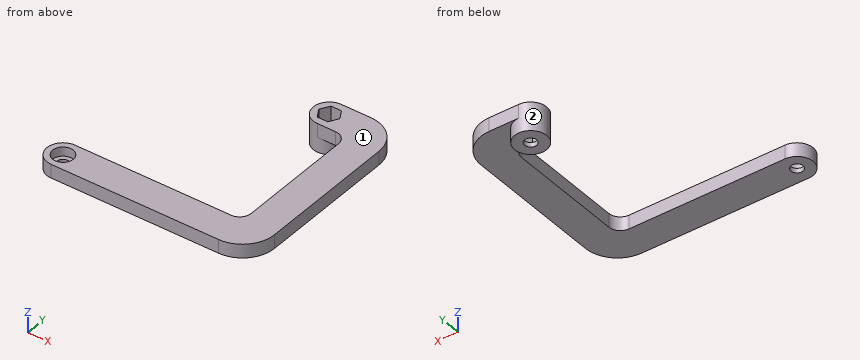
Autodesk Inventor part; units mm, degrees
ref_plane "YZ Plane" through (0, 0, 0) normal (1, 0, 0) x (0, 1, 0)
ref_plane "XZ Plane" through (0, 0, 0) normal (0, 1, 0) x (-1, 0, 0)
ref_plane "XY Plane" through (0, 0, 0) normal (0, 0, 1) x (1, 0, 0)
sketch "Skizze1" plane through (0, 0, 0) normal (0, 0, 1) x (1, 0, 0)
  circle A0 centre (0, 0) radius 2.5
  line L0 (0, 7) -> (13, 7)
  arc A1 (0, 7) -> (0, -7) centre (0, 0) ccw
  circle A2 centre (-60.334, -75) radius 2.5
  line L1 (-60.334, -68) -> (8, -68)
  line L2 (13, -63) -> (13, -12)
  line L3 (27, -7) -> (27, -68)
  line L4 (13, -82) -> (-60.334, -82)
  arc A3 (-60.334, -68) -> (-60.334, -82) centre (-60.334, -75) ccw
  line L5 (20, -82) -> (20, 7) construction
  line L6 (0, 0) -> (-60.334, -75) construction
  line L7 (-60.334, -75) -> (-110.6881, -137.5941) construction
  line L8 (-60.334, -75) -> (20, -75) construction
  circle A4 centre (-60.334, -75) radius 7
  arc A5 (27, -7) -> (13, 7) centre (13, -7) ccw
  arc A6 (13, -82) -> (27, -68) centre (13, -68) ccw
  arc A7 (8, -68) -> (13, -63) centre (8, -63) ccw
  arc A8 (13, -12) -> (8, -7) centre (8, -12) ccw
  circle A9 centre (0, 0) radius 7
  line L9 (8, -7) -> (0, -7)
  line L10 (-2.3094, -4) -> (-4.6188, 0)
  line L11 (-4.6188, 0) -> (-2.3094, 4)
  line L12 (-2.3094, 4) -> (2.3094, 4)
  line L13 (2.3094, 4) -> (4.6188, 0)
  line L14 (4.6188, 0) -> (2.3094, -4)
  line L15 (2.3094, -4) -> (-2.3094, -4)
  point P0 (-60.334, -68)
  point P1 (13, 7)
  point P2 (0, -7)
  point P3 (0, -7)
  dimension "d0" = 5
  dimension "d10" = 75
  dimension "d11" = 14
  dimension "d14" = 176.5899
  dimension "d19" = 20
  dimension "d20" = 7
  dimension "d25" = 5
  dimension "d26" = 14
  dimension "d41" = 8
extrude "Extrusion1" add sketch "Skizze1" along normal blind 6 contours A9 A1 | L0 A5 L3 A6 L4 A4 L1 A7 L2 A8 L9 A9 | A3 A4 | L10 L11 L12 L13 L14 L15
extrude "Extrusion2" add sketch "Skizze1" against normal blind 6.5 contours A9 A1 | L10 L11 L12 L13 L14 L15
sketch "Skizze2" plane through (0, 0, 6) normal (0, 0, 1) x (1, 0, 0)
  circle A0 centre (-60.334, -75) radius 2.5
  circle A1 centre (0, 0) radius 2.5
hole "Bohrung1" at (-60.334, -75, 6) direction (0, 0, -1) diameter 5.3 end through all counterbore diameter 9 counterbore depth 4
sketch "Skizze3" plane through (0, 0, 6) normal (0, 0, 1) x (1, 0, 0)
  circle A0 centre (0, 0) radius 2.5
hole "Bohrung2" at (0, 0, 6) direction (0, 0, -1) diameter 5.3 end through all
extrude "Extrusion3" cut sketch "Skizze1" along normal blind 6 and the other way blind 4.5 contours L10 L11 L12 L13 L14 L15
equation "\"d11\" = 2 * d20"
equation "\"d26\" = 2 * d20"
equation "\"d42\" = d6"
properties part number "Door_Lever2" material "ABS-Kunststoff"
Work out the finished part from the listing and answer in its coordinate system (mm). Face numbers are marked on the shaded views. Coordinates: 2 decimals unless noted, no trailing zeros. Loops run counter-clockwise (first coordinate to the right, second up) from the corner with the lowest first, then second, coordinate; pieces in that order, holes last. Notation, with made-up numbers: (78.25, -9) -> (110.25, -9) arc R23 ccw to (110.25, 11) -> close; hole circle Ø6 at (-34, 12.5). An arc over 180 degrees is marked (long way). Answer as CSV lines item,"result".
Q1. For a pull along Y with two mould halves and no side action, classify the marked faces 1 and 2 as +Y half, -Y half, draft (parallel to the pull), parting line (faces both ways), or undercut.
Findings:
face 1,"draft"
face 2,"undercut"
Q2. Each of these flat-tipped pins is pushed along its axis until it touches: pin 1 (4 mm diameter, centred on x = -39.5, z = 3, fed in from +Y); pin 2 (14.5 mm diameter, centred on x = -60.334, y = -75, fed in from +Z); pin 3 (5 mm diameter, centred on y = -27.5, z = 2, fed in from -X); pin 4 (2.5 mm diameter, centred on x = 2, y = -1, fed in from +Z). Where does it stop, or does it pass through?
Findings:
pin 1,"stops at y = -68"
pin 2,"stops at z = 6"
pin 3,"stops at x = 13"
pin 4,"stops at z = -4.5"
Q3. The part is cut by section A-A on y = -76. Write down the section's boundary in (x, z).
Findings:
outline,"(-67.26, 0) -> (-62.79, 0) -> (-62.79, 2) -> (-64.72, 2) -> (-64.72, 6) -> (-67.26, 6) -> close; (-57.88, 0) -> (24.49, 0) -> (24.49, 6) -> (-55.95, 6) -> (-55.95, 2) -> (-57.88, 2) -> close"
Q4. The part is cut by section B-B on x = -11.5. Write down the section's boundary in (y, z), and give its area (3 significant figures).
Findings:
outline,"(-82, 0) -> (-68, 0) -> (-68, 6) -> (-82, 6) -> close"
area,"84.0 mm²"
Q5. Find the intervals of material crossed by probe 1 along Y at (x, z) = (1, 5.75); probe 2 along Y at (x, z) = (4, 2.5); probe 3 along X at (y, z) = (0, -5.4), in increasing order.
Findings:
probe 1,"y = -82 to -68, -7 to -4, 4 to 7"
probe 2,"y = -82 to -68, -7 to -1.07, 1.07 to 7"
probe 3,"x = -7 to -2.65, 2.65 to 7"
Q6. The part is cut by section C-C on y = -23. Write down the section's boundary in (x, z), and give its area (3 significant figures).
Findings:
outline,"(13, 0) -> (27, 0) -> (27, 6) -> (13, 6) -> close"
area,"84.0 mm²"
